Work out the finished part from the listing and answer in its coordinate system (mm). Face numbers are marked on the shaded views. A direction names the side the tool comes from. Round coordinates to 2 decimals unless told otherwise and drop trailing zeros. Loops run counter-clockwise (first coordinate to the right, second up) from the corner with the lowest first, then second, coordinate; pieces in that order, holes last. Notation, with made-up numbers: (-34.75, -31) - (15.25, -31) arc R26 cw to (15.25, -8) - close; hole circle Ø4 at (-25, 31.25). An arc over 180 degrees is marked (long way). Answer as CSV lines item,"result". Start each with the question number.
Q1. Each of these flat-tipped pins is pushed along its axis until it touches: pin 1 Ø6 at (x, z) = (1, 5.5) entering from +Y; pin 2 Ø2 at (x, y) = (-0.5, 13.5) entering from +Z; pin 3 Ø1.5 at (x, z) = (-6, 4.5) entering from -Y; pin 4 Ø6 at (x, y) = (6, 20.5) entering from +Z. Where does it stop, or does it pass through?
Q2. Straight lines are drawn through the part: L1, parallel to X at y = 20.5, z = 1.5; L2, parallel to Z at x = 0, y = 24.5; L3, parallel to X at y = 15.5, z = 5.25. For each, find the intervals that lie inside material, in ascending order. Write a range as [from, to].
Q3. Section B-B on y = 16.5 is taken. Write down the section's boundary in (x, z).
Q4. Section A-A on x = 2.75 is taken. Write down the section's boundary in (y, z).
Q5. For the marked faces 5, 6 and 7, determine the directions among +Z, -Z, +X, -X, +Y, -Y from which every point of the face is accessible in a straight line to the end or side of a thin tool.
Q6. Section D-D on y = 3.75 is taken. Write down the section's boundary in (x, z), then the cut area to 3 significant figures.
Q7. The mould has two halves that part along Y. Classify the marked faces 1, 2, 3 and 4: +Y half, -Y half, draft (parallel to the pull), parting line (faces both ways), or undercut.
```python
from build123d import *

# Parameters (mm, degrees)
F0_W     = 16
F0_H     = 26.1
F1_DEPTH = 11
F2_R     = 9
F3_DEPTH = 25
F5_DEPTH = 12.5
F6_R     = 4.5
F7_R     = 4.25


# Not quite as in the source:
# - an extrude whose draft closes it to a point is written as a loft to that point


with BuildPart() as f1:
    # F0 (on Top) → F1 (new body)
    with BuildSketch(Plane.XY):
        with Locations((0, 13.05)):
            Rectangle(F0_W, F0_H)
    extrude(amount=F1_DEPTH)

    # F2 (on Top) → F3 (cut)
    with BuildSketch(Plane.XY):
        with Locations((-14.65, 13.05)):
            Circle(F2_R)
        with Locations((14.65, 13.05)):
            Circle(F2_R)
    extrude(amount=F3_DEPTH, mode=Mode.SUBTRACT)

    # F4 (on Right) → F5 (cut, symmetric)
    with BuildSketch(Plane.YZ):
        Polygon((0, 4), (26.1, 11), (0, 11), align=None)
    extrude(amount=F5_DEPTH, both=True, mode=Mode.SUBTRACT)

    # F6
    f6_edges = [f1.edges().sort_by_distance(p)[0] for p in [
        (-8, 26.1, 5.5),
        (-8, 6.985554, 2.93676),
        (-8, 19.114446, 4.56324),
        (-8, 0, 2),
        (8, 0, 2),
        (8, 6.985554, 2.93676),
        (8, 19.114446, 4.56324),
        (8, 26.1, 5.5),
    ]]
    fillet(f6_edges, radius=F6_R)

    # F7 (on face) → F8 section 0
    with BuildSketch(Plane(origin=(0, 26.1, 0), x_dir=(-1, 0, 0), z_dir=(0, 1, 0)), mode=Mode.PRIVATE) as f8_s0:
        with Locations((-2.75, 5.5)):
            Circle(F7_R)
    loft([f8_s0.sketch, Vertex(2.75, 4.2356454321, 5.5)], ruled=True, mode=Mode.SUBTRACT)


solid = f1.part
```
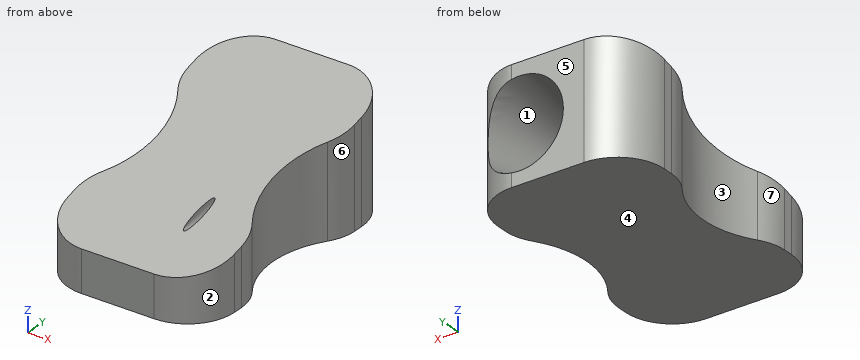
Findings:
1,pin 1,"stops at y = 26.1"
1,pin 2,"stops at z = 7.89"
1,pin 3,"stops at y = 0.4"
1,pin 4,"stops at z = 10.3"
2,L1,"x = [-8, 8]"
2,L2,"z = [0, 2.68], [8.32, 10.57]"
2,L3,"x = [-5.99, 0.57], [4.93, 5.99]"
3,outline,"(-6.34, 0) - (6.34, 0) - (6.34, 8.43) - (-6.34, 8.43) - close; hole circle Ø4.77 at (2.75, 5.5)"
4,outline,"(0, 0) - (26.1, 0) - (26.1, 1.25) - (5.02, 5.35) - (0, 4) - close; (9.17, 6.46) - (26.1, 9.75) - (26.1, 11) - close"
5,face 5,"+Z, -Z, +X, -X, +Y"
5,face 6,"+Z, -Z, +X"
5,face 7,"+Z, -Z, -X"
6,outline,"(-7.94, 0) - (7.94, 0) - (7.94, 5.01) - (-7.94, 5.01) - close"
6,area,"79.5 mm^2"
7,face 1,"+Y half"
7,face 2,"-Y half"
7,face 3,"undercut"
7,face 4,"draft"
